Part model, mm, in its own coordinate system. A direction names the side the tool comes from. Coordinates: 2 decimals unless noted, no trailing zeros. Order: outer loops, then holes, each group sorted by start corner. A loop starts at its lowest first (then second) coordinate and runs counter-clockwise, first axis right, second up.
from build123d import *

# Parameters (mm, degrees)
SKETCH1_W                = 152.4
SKETCH1_H                = 152.4
BOSS_EXTRUDE1_DEPTH      = 8.466666667
BOSS_EXTRUDE3_DEPTH      = 101.6
SKETCH4_R                = 5.006944118
BOSS_EXTRUDE4_DEPTH      = 6.35
CUT_EXTRUDE1_REACH       = 205.785
SKETCH6_W                = 84.1375
SKETCH6_H                = 30.46777391
FILLET1_R                = 12.54
CIRPATTERN3_COUNT        = 3
FILLET1_OF_CIRPATTERN3_R = 12.54
SKETCH8_R                = 3.175
CUT_EXTRUDE2_DEPTH       = 6.35
SKETCH9_R                = 15.793040305
CUT_EXTRUDE4_DEPTH       = 153.593412515


with BuildPart() as part:
    # Sketch1 → Boss-Extrude1 (new body)
    with BuildSketch(Plane(origin=(0, 0, 0), x_dir=(1, 0, 0), z_dir=(0, 1, 0))):
        with Locations((0, -0.122388871)):
            Rectangle(SKETCH1_W, SKETCH1_H)
    extrude(amount=BOSS_EXTRUDE1_DEPTH)

    # Sketch3 → Boss-Extrude3 (add)
    with BuildSketch(Plane(origin=(0, 8.466666667, 0), x_dir=(1, 0, 0), z_dir=(0, 1, 0))):
        with BuildLine():
            ThreePointArc((-58.918716059, 39.286110084), (-65.909577408, 37.544355622), (-63.922550345, 30.619214868))
            ThreePointArc((-63.922550345, 30.619214868), (-61.573436607, 35.040883563), (-58.918716059, 39.286110084))
        make_face()
        with BuildLine():
            ThreePointArc((-58.918716059, 39.286110084), (-61.573436607, 35.040883563), (-63.922550345, 30.619214868))
            ThreePointArc((-63.922550345, 30.619214868), (-58.993939739, 30.749533507), (-56.566492489, 35.040883563))
            ThreePointArc((-56.566492489, 35.040883563), (-57.193851762, 37.467553294), (-58.918716059, 39.286110084))
        make_face()
        with BuildLine():
            Line((45.987944587, 60.142290401), (-46.087055413, 60.142290401))
            ThreePointArc((-46.087055413, 60.142290401), (-65.972845658, 37.580883563), (-75.568702003, 9.078580617))
            Line((-75.568702003, 9.078580617), (-29.531202003, -70.660708437))
            ThreePointArc((-29.531202003, -70.660708437), (-18.268592558, -74.38917131), (-6.563445111, -76.322388871))
            Line((-6.563445111, -76.322388871), (-1.471511547, -76.322388871))
            ThreePointArc((-1.471511547, -76.322388871), (-4.113530257, -74.446258004), (-5.053389698, -71.345162371))
            ThreePointArc((-5.053389698, -71.345162371), (-15.708360105, -69.77438362), (-26.003436632, -66.610977296))
            Line((-26.003436632, -66.610977296), (-70.297649271, 10.108849476))
            ThreePointArc((-70.297649271, 10.108849476), (-67.889701246, 20.606350444), (-63.922550345, 30.619214868))
            ThreePointArc((-63.922550345, 30.619214868), (-65.909577408, 37.544355622), (-58.918716059, 39.286110084))
            ThreePointArc((-58.918716059, 39.286110084), (-52.230896554, 47.728195757), (-44.343768052, 55.062290401))
            Line((-44.343768052, 55.062290401), (44.244657227, 55.062290401))
            ThreePointArc((44.244657227, 55.062290401), (52.131785728, 47.728195757), (58.819605234, 39.286110084))
            ThreePointArc((58.819605234, 39.286110084), (63.900995513, 39.420468408), (66.481269899, 35.040883563))
            ThreePointArc((66.481269899, 35.040883563), (65.765675838, 32.461386695), (63.823439519, 30.619214868))
            ThreePointArc((63.823439519, 30.619214868), (67.790590421, 20.606350444), (70.198538446, 10.108849476))
            Line((70.198538446, 10.108849476), (25.904325806, -66.610977296))
            ThreePointArc((25.904325806, -66.610977296), (15.60924928, -69.77438362), (4.954278873, -71.345162371))
            ThreePointArc((4.954278873, -71.345162371), (4.956611187, -71.433369756), (4.957388705, -71.521604544))
            ThreePointArc((4.957388705, -71.521604544), (3.962248689, -74.517421169), (1.372400721, -76.322388871))
            Line((1.372400721, -76.322388871), (6.464334286, -76.322388871))
            ThreePointArc((6.464334286, -76.322388871), (18.169481733, -74.38917131), (29.432091177, -70.660708437))
            Line((29.432091177, -70.660708437), (75.469591177, 9.078580617))
            ThreePointArc((75.469591177, 9.078580617), (65.873734833, 37.580883563), (45.987944587, 60.142290401))
        make_face()
        with BuildLine():
            ThreePointArc((4.954278873, -71.345162371), (-0.049555413, -66.514660427), (-5.053389698, -71.345162371))
            ThreePointArc((-5.053389698, -71.345162371), (-0.049555413, -71.521604544), (4.954278873, -71.345162371))
        make_face()
        with BuildLine():
            ThreePointArc((-5.053389698, -71.345162371), (-4.113530257, -74.446258004), (-1.471511547, -76.322388871))
            Line((-1.471511547, -76.322388871), (1.372400721, -76.322388871))
            ThreePointArc((1.372400721, -76.322388871), (3.962248689, -74.517421169), (4.957388705, -71.521604544))
            ThreePointArc((4.957388705, -71.521604544), (4.956611187, -71.433369756), (4.954278873, -71.345162371))
            ThreePointArc((4.954278873, -71.345162371), (-0.049555413, -71.521604544), (-5.053389698, -71.345162371))
        make_face()
        with BuildLine():
            ThreePointArc((58.819605234, 39.286110084), (57.13818498, 32.537411504), (63.823439519, 30.619214868))
            ThreePointArc((63.823439519, 30.619214868), (61.474325782, 35.040883563), (58.819605234, 39.286110084))
        make_face()
        with BuildLine():
            ThreePointArc((58.819605234, 39.286110084), (61.474325782, 35.040883563), (63.823439519, 30.619214868))
            ThreePointArc((63.823439519, 30.619214868), (65.765675838, 32.461386695), (66.481269899, 35.040883563))
            ThreePointArc((66.481269899, 35.040883563), (63.900995513, 39.420468408), (58.819605234, 39.286110084))
        make_face()
    extrude(amount=BOSS_EXTRUDE3_DEPTH)

    # Sketch4 → Boss-Extrude4 (add)
    with BuildSketch(Plane(origin=(0, 110.066666667, 0), x_dir=(1, 0, 0), z_dir=(0, 1, 0))):
        with Locations(Location((61.474325782, 35.040883563, 0), (0, 0, 122.019492362))):
            Circle(SKETCH4_R)
        with Locations(Location((0.128367161, -70.759732709, 0), (0, 0, 171.336111326))):
            Circle(SKETCH4_R)
        with Locations(Location((-61.601057978, 34.817609153, 0), (0, 0, 354.23508657))):
            Circle(SKETCH4_R)
    extrude(amount=BOSS_EXTRUDE4_DEPTH)

    # Sketch6 → Cut-Extrude1 (cut, up to next)
    with BuildSketch(Plane(origin=(-52.74538578, 0, 30.452562679), x_dir=(0.5, 0, 0.8660254037844386), z_dir=(-0.8660254037844387, 0, 0.5000000000000001)), mode=Mode.PRIVATE) as cut_extrude1_sk1:
        with Locations((0.269593494, 29.172106293)):
            Rectangle(SKETCH6_W, SKETCH6_H)
    cut_extrude1_tool1 = extrude(cut_extrude1_sk1.sketch, amount=-CUT_EXTRUDE1_REACH, mode=Mode.PRIVATE) & part.part
    cut_extrude1 = cut_extrude1_tool1.solids().sort_by_distance((-52.610589, 29.172106, 30.686037))[0]
    add(cut_extrude1, mode=Mode.SUBTRACT)

    # Fillet1
    fillet1_edges = [part.edges().sort_by_distance(p)[0] for p in [
        (-29.376509507, 44.405993248, 65.848643698),
        (-29.376509507, 13.938219338, 65.848643698),
        (-71.445259507, 13.938219338, -7.016568713),
        (-71.445259507, 44.405993248, -7.016568713),
    ]]
    fillet(fillet1_edges, radius=FILLET1_R)

    # CirPattern3: Cut-Extrude1; each copy of Cut-Extrude1 runs up to whatever stops it at its own place
    cirpattern3_before = part.part  # the part as the pattern finds it: every copy runs up to it
    cirpattern3_cut_extrude1_long = extrude(cut_extrude1_sk1.sketch, amount=-CUT_EXTRUDE1_REACH, mode=Mode.PRIVATE)
    cirpattern3_cut_extrude1_tool1 = cirpattern3_cut_extrude1_long.rotate(Axis((0, 0, 0), (0, 1, 0)), 1 * 360 / CIRPATTERN3_COUNT) & cirpattern3_before
    add(cirpattern3_cut_extrude1_tool1.solids().sort_by_distance((52.880182, 29.172106, 30.219088))[0], mode=Mode.SUBTRACT)
    cirpattern3_cut_extrude1_tool2 = cirpattern3_cut_extrude1_long.rotate(Axis((0, 0, 0), (0, 1, 0)), 2 * 360 / CIRPATTERN3_COUNT) & cirpattern3_before
    add(cirpattern3_cut_extrude1_tool2.solids().sort_by_distance((-0.269593, 29.172106, -60.905125))[0], mode=Mode.SUBTRACT)

    # Fillet1 of CirPattern3
    fillet1_of_cirpattern3_edges = [part.edges().sort_by_distance(p)[0] for p in [
        (71.714853001, 44.405993248, -7.483518341),
        (71.714853001, 13.938219338, -7.483518341),
        (29.646103001, 13.938219338, 65.38169407),
        (29.646103001, 44.405993248, 65.38169407),
        (-42.338343494, 44.405993248, -58.365125357),
        (-42.338343494, 13.938219338, -58.365125357),
        (41.799156506, 13.938219338, -58.365125357),
        (41.799156506, 44.405993248, -58.365125357),
    ]]
    fillet(fillet1_of_cirpattern3_edges, radius=FILLET1_OF_CIRPATTERN3_R)

    # Sketch8 → Cut-Extrude2 (cut)
    with BuildSketch(Plane(origin=(0, 0, 0), x_dir=(-1, 0, 0), z_dir=(0, -1, 0))):
        with Locations(Location((63.5, -38.222388871, 0), (0, 0, 90))):
            Circle(SKETCH8_R)
        with Locations(Location((38.1, -63.622388871, 0), (0, 0, 90))):
            Circle(SKETCH8_R)
        with Locations(Location((-63.5, -38.222388871, 0), (0, 0, 270))):
            Circle(SKETCH8_R)
        with Locations(Location((-38.1, -63.622388871, 0), (0, 0, 270))):
            Circle(SKETCH8_R)
        with Locations(Location((63.5, 37.977611129, 0), (0, 0, 90))):
            Circle(SKETCH8_R)
        with Locations(Location((38.1, 63.377611129, 0), (0, 0, 90))):
            Circle(SKETCH8_R)
        with Locations(Location((-38.1, 63.377611129, 0), (0, 0, 90))):
            Circle(SKETCH8_R)
        with Locations(Location((-63.5, 37.977611129, 0), (0, 0, 90))):
            Circle(SKETCH8_R)
    extrude(amount=-CUT_EXTRUDE2_DEPTH, mode=Mode.SUBTRACT)

    # Sketch9 → Cut-Extrude4 (cut, through all)
    with BuildSketch(Plane(origin=(0, 8.466666667, 0), x_dir=(1, 0, 0), z_dir=(0, 1, 0))):
        with Locations(Location((0, 0, 0), (0, 0, 270))):
            Circle(SKETCH9_R)
    extrude(amount=-CUT_EXTRUDE4_DEPTH, mode=Mode.SUBTRACT)


solid = part.part
Q1. Cut at C-C on z = 21. Write the cut outline in (x, y), and give its area (3 significant figures).
Results list:
outline: (-76.2, 0) - (76.2, 0) - (76.2, 8.47) - (58.1, 8.47) - (58.1, 13.94) - (52.24, 13.94) - (52.24, 8.47) - (-52.34, 8.47) - (-52.34, 13.94) - (-58.2, 13.94) - (-58.2, 8.47) - (-76.2, 8.47) - close; (-58.2, 44.41) - (-52.34, 44.41) - (-52.34, 110.07) - (-58.2, 110.07) - close; (52.24, 44.41) - (58.1, 44.41) - (58.1, 110.07) - (52.24, 110.07) - close
area: 2,120 mm2
Q2. Cut at B-B on x = 0. Write the cut outline in (y, z).
Results list:
outline: (0, -76.08) - (8.47, -76.08) - (8.47, -60.14) - (13.94, -60.14) - (13.94, -55.06) - (8.47, -55.06) - (8.47, -15.79) - (0, -15.79) - close; (0, 15.79) - (8.47, 15.79) - (8.47, 66.51) - (110.07, 66.51) - (110.07, 65.75) - (116.42, 65.75) - (116.42, 75.77) - (110.07, 75.77) - (110.07, 76.32) - (0, 76.32) - close; (44.41, -60.14) - (110.07, -60.14) - (110.07, -55.06) - (44.41, -55.06) - close
Q3. Pin check, flat tips, straight feed: pin 1 Ø3 at (x, z) = (5, 19.5) entering from -Y; pin 2 Ø12 at (y, z) = (101, -57.5) entering from +X; pin 3 Ø5 at (x, z) = (-35.5, 14.5) entering from +Y; pin 4 Ø3 at (y, z) = (60, -13.5) entering from +X. Stop position of each tip, or through.
Results list:
pin 1: stops at y = 0
pin 2: stops at x = 55.56
pin 3: stops at y = 8.47
pin 4: stops at x = 75.04
Q4. Which spindle directions (+Z, -Z, +X, -X, +Y, -Y) get a long thin tool onto all of the face, cutting with end or side? Do faces 1 (the face through (-71.476, 29.134, -6.999)), 2 (the face through (35.954, 3.131, 61.282)), 3 (the face through (-38.6, 40.8, -57.6)). Say none if no direction does.
Results list:
face 1: +Z
face 2: -Y
face 3: -Z
Q5. Mould opens along X. For faces 4 (the face through (-31.231, 40.83, 62.565)), 5 (the face through (-1, 70, -55.062)), 6 (the face through (0, 116.417, 71)) say: pulls with the +X half, pulls with the -X half, needs draft (parallel to the pull), parting line crosses it, or undercut.
Results list:
face 4: pulls with the -X half
face 5: undercut
face 6: needs draft
Q6. Cut at A-A on y = 16. Count the separate pieces of the cut face and the enclosed holes in it, and give its area (3 significant figures).
Results list:
separate pieces: 3
enclosed holes: 0
area: 1,250 mm2
Q7. Wall check: line 1 along Z through (x, y) = (-38, 4); line 2 along Z through (x, y) = (-63, 4); line 3 along X through (y, z) = (2.25, 0). Give the ranges that are in metal, low to high.
Results list:
line 1: z = -76.08 to -66.55, -60.2 to 60.45, 66.8 to 76.32
line 2: z = -76.08 to -41.11, -34.84 to 35.09, 41.36 to 76.32
line 3: x = -76.2 to -15.79, 15.79 to 76.2
